```python
from build123d import *

# Parameters (mm, degrees)
CYLINDER009_R     = 0.8
CYLINDER009_DEPTH = 20
CYLINDER010_R     = 0.8
CYLINDER010_DEPTH = 20
CYLINDER011_R     = 0.8
CYLINDER011_DEPTH = 20
CYLINDER008_R     = 0.8
CYLINDER008_DEPTH = 20
CYLINDER005_R     = 0.34
CYLINDER005_DEPTH = 100
CYLINDER006_R     = 0.34
CYLINDER006_DEPTH = 100
CYLINDER007_R     = 0.34
CYLINDER007_DEPTH = 100
CYLINDER004_R     = 0.34
CYLINDER004_DEPTH = 100
CYLINDER002_R     = 4.75
CYLINDER002_DEPTH = 0.5
CYLINDER003_R     = 4.75
CYLINDER003_DEPTH = 0.5
BOX008_W          = 18
BOX008_H          = 9.5
BOX008_DEPTH      = 0.5
BOX004_W          = 40
BOX004_H          = 1
BOX004_DEPTH      = 2.5
CYLINDER001_R     = 2
CYLINDER001_DEPTH = 20
BOX002_W          = 40
BOX002_H          = 42
BOX002_DEPTH      = 6
BOX001_W          = 42
BOX001_H          = 44
BOX001_DEPTH      = 7
BOX003_W          = 40
BOX003_H          = 1
BOX003_DEPTH      = 2.5


with BuildPart() as zylinder009:
    # Cylinder009 → Cylinder009 (new body)
    with BuildSketch(Plane(origin=(2.5, 2.5, -10), x_dir=(1, 0, 0), z_dir=(0, 0, 1))):
        Circle(CYLINDER009_R)
    extrude(amount=CYLINDER009_DEPTH)


with BuildPart() as zylinder010:
    # Cylinder010 → Cylinder010 (new body)
    with BuildSketch(Plane(origin=(37.5, 39.5, -10), x_dir=(1, 0, 0), z_dir=(0, 0, 1))):
        Circle(CYLINDER010_R)
    extrude(amount=CYLINDER010_DEPTH)


with BuildPart() as zylinder011:
    # Cylinder011 → Cylinder011 (new body)
    with BuildSketch(Plane(origin=(2.5, 39.5, -10), x_dir=(1, 0, 0), z_dir=(0, 0, 1))):
        Circle(CYLINDER011_R)
    extrude(amount=CYLINDER011_DEPTH)


with BuildPart() as compound005:
    # Cylinder008 → Cylinder008 (new body)
    with BuildSketch(Plane(origin=(37.5, 2.5, -10), x_dir=(1, 0, 0), z_dir=(0, 0, 1))):
        Circle(CYLINDER008_R)
    extrude(amount=CYLINDER008_DEPTH)

    # Compound005: union Zylinder009, Zylinder010, Zylinder011
    add(zylinder009.part)
    add(zylinder010.part)
    add(zylinder011.part)


with BuildPart() as zylinder005:
    # Cylinder005 → Cylinder005 (new body)
    with BuildSketch(Plane(origin=(18.24, 28, -50), x_dir=(1, 0, 0), z_dir=(0, 0, 1))):
        Circle(CYLINDER005_R)
    extrude(amount=CYLINDER005_DEPTH)


with BuildPart() as zylinder006:
    # Cylinder006 → Cylinder006 (new body)
    with BuildSketch(Plane(origin=(36, 14.5, -50), x_dir=(1, 0, 0), z_dir=(0, 0, 1))):
        Circle(CYLINDER006_R)
    extrude(amount=CYLINDER006_DEPTH)


with BuildPart() as zylinder007:
    # Cylinder007 → Cylinder007 (new body)
    with BuildSketch(Plane(origin=(36, 27.5, -50), x_dir=(1, 0, 0), z_dir=(0, 0, 1))):
        Circle(CYLINDER007_R)
    extrude(amount=CYLINDER007_DEPTH)


with BuildPart() as m1tapholes:
    # Cylinder004 → Cylinder004 (new body)
    with BuildSketch(Plane(origin=(18.24, 14, -50), x_dir=(1, 0, 0), z_dir=(0, 0, 1))):
        Circle(CYLINDER004_R)
    extrude(amount=CYLINDER004_DEPTH)

    # Compound002: union Zylinder005, Zylinder006, Zylinder007
    add(zylinder005.part)
    add(zylinder006.part)
    add(zylinder007.part)


with BuildPart() as zylinder002:
    # Cylinder002 → Cylinder002 (new body)
    with BuildSketch(Plane(origin=(27.75, 25.75, -4.4), x_dir=(1, 0, 0), z_dir=(0, 0, 1))):
        Circle(CYLINDER002_R)
    extrude(amount=CYLINDER002_DEPTH)


with BuildPart() as zylinder003:
    # Cylinder003 → Cylinder003 (new body)
    with BuildSketch(Plane(origin=(27.75, 16.25, -4.4), x_dir=(1, 0, 0), z_dir=(0, 0, 1))):
        Circle(CYLINDER003_R)
    extrude(amount=CYLINDER003_DEPTH)


with BuildPart() as fusion002:
    # Box008 → Box008 (new body)
    with BuildSketch(Plane(origin=(23, 16.25, -4.4), x_dir=(1, 0, 0), z_dir=(0, 0, 1))):
        with Locations((9, 4.75)):
            Rectangle(BOX008_W, BOX008_H)
    extrude(amount=BOX008_DEPTH)

    # Fusion002: union Zylinder002, Zylinder003
    add(zylinder002.part)
    add(zylinder003.part)


with BuildPart() as obj1:
    # Box004 → Box004 (new body)
    with BuildSketch(Plane(origin=(0, 41, -3.4), x_dir=(1, 0, 0), z_dir=(0, 0, 1))):
        with Locations((20, 0.5)):
            Rectangle(BOX004_W, BOX004_H)
    extrude(amount=BOX004_DEPTH)


with BuildPart() as zylinder001:
    # Cylinder001 → Cylinder001 (new body)
    with BuildSketch(Plane(origin=(30, 21, -10), x_dir=(1, 0, 0), z_dir=(0, 0, 1))):
        Circle(CYLINDER001_R)
    extrude(amount=CYLINDER001_DEPTH)


with BuildPart() as obj2:
    # Box002 → Box002 (new body)
    with BuildSketch(Plane.XY.offset(-3.4)):
        with Locations((20, 21)):
            Rectangle(BOX002_W, BOX002_H)
    extrude(amount=BOX002_DEPTH)


with BuildPart() as cut002:
    # Box001 → Box001 (new body)
    with BuildSketch(Plane(origin=(-1, -1, -4.4), x_dir=(1, 0, 0), z_dir=(0, 0, 1))):
        with Locations((21, 22)):
            Rectangle(BOX001_W, BOX001_H)
    extrude(amount=BOX001_DEPTH)

    # Cut001: cut obj2
    add(obj2.part, mode=Mode.SUBTRACT)

    # Cut002: cut Zylinder001
    add(zylinder001.part, mode=Mode.SUBTRACT)


with BuildPart() as upperpart:
    # Box003 → Box003 (new body)
    with BuildSketch(Plane.XY.offset(-3.4)):
        with Locations((20, 0.5)):
            Rectangle(BOX003_W, BOX003_H)
    extrude(amount=BOX003_DEPTH)

    # Fusion: union obj1, Cut002
    add(obj1.part)
    add(cut002.part)

    # Cut004: cut Fusion002
    add(fusion002.part, mode=Mode.SUBTRACT)

    # Cut005: cut M1TapHoles
    add(m1tapholes.part, mode=Mode.SUBTRACT)

    # Cut007: cut Compound005
    add(compound005.part, mode=Mode.SUBTRACT)


solid = upperpart.part
```
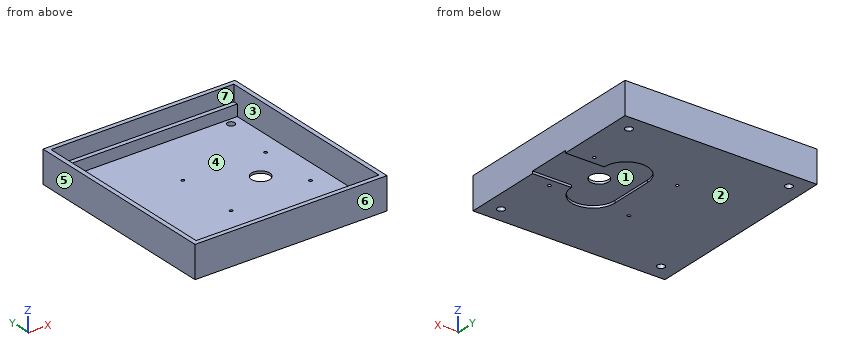
Model file for the job. Use its own axes, mm. Face numbers are marked on the shaded views. A direction names the side the tool comes from. Give positions to 0.01 mm unless a question says otherwise; leave off trailing zeros. Loops run counter-clockwise (first coordinate to the right, second up) from the corner with the lowest first, then second, coordinate; pieces in that order, holes last. Notation, with made-up numbers: M 19.25,-1.75 L 25.25,-1.75 A14 ccw 25.25,12.25 Z; hole C 85,-27.5 d5. An arc over 180 degrees is marked long. Use one line per item in the form item = value.
Item 1: Two-plate mould, pull along Y, no slides. Class the marked faces 4, 5, 6 and 7: released by +Y, released by -Y, zero draft, split by the parting line, or undercut.
Filled in:
face_4 = undercut
face_5 = zero draft
face_6 = released by -Y
face_7 = undercut
Item 2: Drill centre lines: L1, parallel to X at y = 2.5, z = -4; L2, parallel to Y at x = 18.24, z = -3.85; L3, parallel to Y at x = 38.5, z = 0.5. Where is each one in solid material? Low to high.
Filled in:
L1 = -1 to 1.7, 3.3 to 36.7, 38.3 to 41
L2 = -1 to 13.66, 14.34 to 27.66, 28.34 to 43
L3 = -1 to 0, 42 to 43
Item 3: Flat gauge pins, fed straight in: pin 1 Ø1.4 at (x, y) = (37.5, 39.5) entering from -Z; pin 2 Ø3 at (x, y) = (27.5, 34.5) entering from +Z; pin 3 Ø5 at (x, y) = (30, 21) entering from -Z. Where does each tip first touch, or does it go through?
Filled in:
pin_1 = through
pin_2 = -3.4
pin_3 = -3.9
Item 4: Slice it at D-D on z = -1.75. List the corners of the cut face in (x, y).
Filled in:
outline = M -1,-1 L 41,-1 L 41,43 L -1,43 Z; hole M 0,1 L 40,1 L 40,41 L 0,41 Z
Item 5: Slice it at C-C on x = 20.5. List the corners of the cut face in (y, z), and give its area (3 significant figures).
Filled in:
outline = M -1,-4.4 L 43,-4.4 L 43,2.6 L 42,2.6 L 42,-0.9 L 41,-0.9 L 41,-3.4 L 1,-3.4 L 1,-0.9 L 0,-0.9 L 0,2.6 L -1,2.6 Z
area = 61.0 mm^2
Item 6: Which spindle directions (+Z, -Z, +X, -X, +Y, -Y) get a long thin tool onto all of the face, cutting with end or side? Do the marked faces 1, 2 and 3. Say none if no direction does.
Filled in:
face_1 = -Z
face_2 = -Z, +X, -X, +Y, -Y
face_3 = +Z
Item 7: Slice it at B-B on z = 1. List the corners of the cut face in (x, y).
Filled in:
outline = M -1,-1 L 41,-1 L 41,43 L -1,43 Z; hole M 0,0 L 40,0 L 40,42 L 0,42 Z
Item 8: Slice it at A-A on y = 2.5. List the corners of the cut face in (x, z), and give its area (3 significant figures).
Filled in:
outline = M -1,-4.4 L 1.7,-4.4 L 1.7,-3.4 L 0,-3.4 L 0,2.6 L -1,2.6 Z; M 3.3,-4.4 L 36.7,-4.4 L 36.7,-3.4 L 3.3,-3.4 Z; M 38.3,-4.4 L 41,-4.4 L 41,2.6 L 40,2.6 L 40,-3.4 L 38.3,-3.4 Z
area = 50.8 mm^2
